from build123d import *

# Parameters (mm, degrees)
CHAMFER1_SIZE      = 0.25
CUT_EXTRUDE1_START = -1.4000001
CUT_EXTRUDE1_DEPTH = 1.4000001


with BuildPart() as part:
    # Sketch2 → Revolve1 (revolve)
    with BuildSketch(Plane(origin=(0, 0, 0), x_dir=(0, 0, -1), z_dir=(1, 0, 0)), mode=Mode.PRIVATE) as revolve1_sk:
        with BuildLine():
            Line((8, 0), (8, 1.5))
            Line((8, 1.5), (0, 1.5))
            Line((0, 1.5), (0, 2.75))
            Line((0, 2.75), (-0.3, 2.75))
            ThreePointArc((-0.3, 2.75), (-1.39323202, 2.363223225), (-2, 1.375))
            Line((-2, 1.375), (-2, 0))
            Line((-2, 0), (8, 0))
        make_face()
    revolve(revolve1_sk.sketch.rotate(Axis((0, 0, 14.771903323), (0, 0, -1)), 90), axis=Axis((0, 0, 14.771903323), (0, 0, -1)))

    # Chamfer1
    chamfer1_edges = [part.edges().sort_by_distance(p)[0] for p in [
        (-1.5, 0, -8),
    ]]
    chamfer(chamfer1_edges, length=CHAMFER1_SIZE)

    # Sketch3 → Cut-Revolve1 (revolve, cut)
    with BuildSketch(Plane(origin=(0, 0, 0), x_dir=(0, 0, -1), z_dir=(1, 0, 0)), mode=Mode.PRIVATE) as cut_revolve1_sk:
        Polygon((-2, 0), (-2, 1), (-0.6, 1), (-0.022649731, 0), align=None)
    revolve(cut_revolve1_sk.sketch.rotate(Axis((0, 0, 1.261909675), (0, 0, -1)), 90), axis=Axis((0, 0, 1.261909675), (0, 0, -1)), mode=Mode.SUBTRACT)

    # Cut-Extrude1: read off the stored shape, not the designer's step
    # Cut-Extrude1 outline → Cut-Extrude1 (cut)
    with BuildSketch(Plane.XY.offset(2).offset(CUT_EXTRUDE1_START)):
        with BuildLine():
            Line((1, 0), (1, 0.577350269))
            Line((1, 0.577350269), (0.500019222, 0.866014306))
            ThreePointArc((0.500019222, 0.866014306), (0.866030953, 0.499990389), (1, 0))
        make_face()
        with BuildLine():
            ThreePointArc((-0.500019222, 0.866014306), (0, 1), (0.500019222, 0.866014306))
            Line((0.500019222, 0.866014306), (0, 1.154700538))
            Line((0, 1.154700538), (-0.500019222, 0.866014306))
        make_face()
        with BuildLine():
            Line((1, -0.577350269), (1, 0))
            ThreePointArc((1, 0), (0.866030953, -0.499990389), (0.500019222, -0.866014306))
            Line((0.500019222, -0.866014306), (1, -0.577350269))
        make_face()
        with BuildLine():
            ThreePointArc((-1, 0), (-0.866030953, 0.499990389), (-0.500019222, 0.866014306))
            Line((-0.500019222, 0.866014306), (-1, 0.577350269))
            Line((-1, 0.577350269), (-1, 0))
        make_face()
        with BuildLine():
            Line((0, -1.154700538), (0.500019222, -0.866014306))
            ThreePointArc((0.500019222, -0.866014306), (0, -1), (-0.500019222, -0.866014306))
            Line((-0.500019222, -0.866014306), (0, -1.154700538))
        make_face()
        with BuildLine():
            ThreePointArc((-0.500019222, -0.866014306), (-0.866030953, -0.499990389), (-1, 0))
            Line((-1, 0), (-1, -0.577350269))
            Line((-1, -0.577350269), (-0.500019222, -0.866014306))
        make_face()
    extrude(amount=CUT_EXTRUDE1_DEPTH, mode=Mode.SUBTRACT)

    # Cut-Extrude1 2 outline → Cut-Extrude1 2 (revolve)
    with BuildSketch(Plane.XZ):
        Polygon((1.154700598, 0.689316432), (0.999999957, 0.599999975), (1.154700538, 0.5999999), align=None)
    revolve(axis=Axis((0, 0, 0), (0, 0, 1)))


solid = part.part
Can you work these out from the model? Positions are in its coordinate system, mm. A direction names the side the tool comes from. Give positions to 0.01 mm unless a question says otherwise; leave off trailing zeros. Order: outer loops, then holes, each group sorted by start corner. A loop starts at its lowest first (then second) coordinate and runs counter-clockwise, first axis right, second up. Notation, with made-up numbers: M 25.5,-7.75 L 35.5,-7.75 A28 ccw 35.5,19.25 Z; hole C 39,61 d2. An arc over 180 degrees is marked long. One line per question, with ' | ' between items.
Item 1: We'd pull the mould along Y, two halves only. Please class faces 4 (the face through (0, 0, -8)), 5 (the face through (-1, 0, 1)), 6 (the face through (1.43, -0.45, -3.82)): released by +Y, released by -Y, zero draft, split by the parting line, or undercut.
Answer block:
face 4: zero draft | face 5: undercut | face 6: split by the parting line
Item 2: Please list where these lines run through material, in increasing order: L1, parallel to X at y = -0.95, z = 1; L2, parallel to Y at x = 1.8, z = 1; L3, parallel to Z at x = -1.7, y = -1.9.
Answer block:
L1: x = -2.42 to -0.35, 0.35 to 2.42 | L2: y = -1.88 to 1.88 | L3: z = 0 to 1.11
Item 3: I'm going to push flat-ended pins straight in: pin 1 Ø2 at (x, z) = (1, 1) entering from +Y; pin 2 Ø1 at (x, z) = (-0.5, -5.5) entering from -Y; pin 3 Ø1 at (x, z) = (-1.5, 0) entering from -Y. Where does each tip first touch, or does it pass through?
Answer block:
pin 1: stops at y = 2.74 | pin 2: stops at y = -1.5 | pin 3: stops at y = -2.56
Item 4: Suppose I cut it at A-A, the plane z = -3.5. Write out the boundary of the cut face in (x, y), then the cut area to 3 significant figures.
Answer block:
outline: C 0,0 d3 | area: 7.07 mm2
Item 5: For faces 1 (the face through (-1.2, 1.2, 0)), 2 (the face through (1.27, 2.44, 0.15)), 3 (the face through (1, 0, 1)), which set-ups out of +Z, -Z, +X, -X, +Y, -Y let a thin tool reach every point of the face, with its end or its side?
Answer block:
face 1: -Z | face 2: +Z, -Z | face 3: +Z
